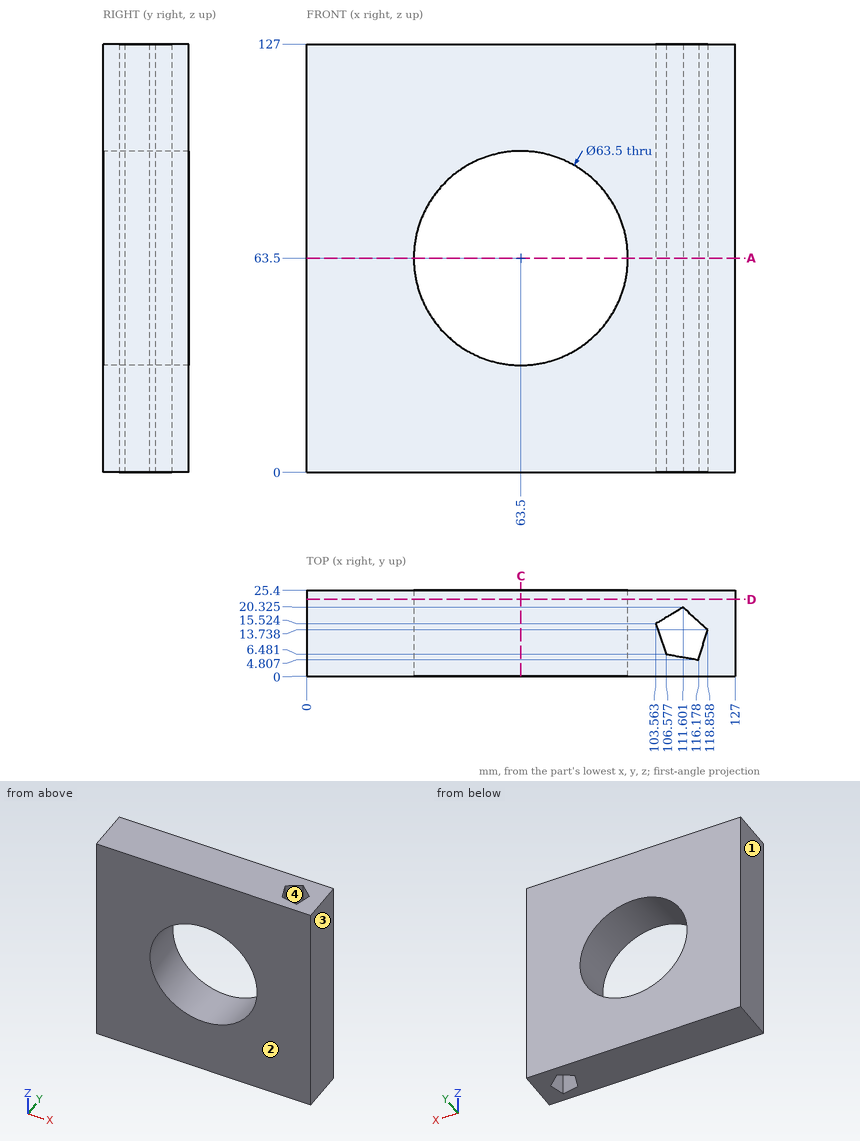
Part print with two shaded views. Sizes in mm from the minimum x, y, z corner. Give positions to 0.01 mm unless a question says otherwise; leave off trailing zeros. Order: outer loops, then holes, each group sorted by start corner. A loop starts at its lowest first (then second) coordinate and runs counter-clockwise, first axis right, second up.
(1) Mould opens along X. For the marked faces 1, 2, 3 and 4 say: released by +X, released by -X, zero draft, split by the parting line, or undercut.
(2) Saw through at D-D, the plane y = 22.75. Give the cut face in (x, z).
(3) Saw through at C-C, the plane x = 63.5. Give the cut face in (y, z), then the cut area to 3 significant figures.
(4) Drill centre lines: L1, parallel to X at y = 14.5, z = 52 (1 decimal); L2, parallel to Z at x = 63.5, y = 15; L3, parallel to X at y = 11, z = 58 (1 decimal). Where is each one in solid material? Low to high.
(5) Saw through at A-A, the plane z = 63.5. State how many separate pieces and enclosed holes the cut face has, then the cut area to 3 significant figures.
Results found:
1. face 1: released by -X
1. face 2: zero draft
1. face 3: released by +X
1. face 4: undercut
2. outline: (0, 0) - (127, 0) - (127, 127) - (0, 127) - close; hole circle Ø63.5 at (63.5, 63.5)
3. outline: (0, 0) - (25.4, 0) - (25.4, 31.75) - (0, 31.75) - close; (0, 95.25) - (25.4, 95.25) - (25.4, 127) - (0, 127) - close
3. area: 1,610 mm2
4. L1: x = 0 to 33.9, 93.1 to 103.9, 118 to 127
4. L2: z = 0 to 31.75, 95.25 to 127
4. L3: x = 0 to 32.2, 94.8 to 105.1, 118 to 127
5. separate pieces: 2
5. enclosed holes: 1
5. area: 1,460 mm2
